from build123d import *

# Parameters (mm, degrees)
Y_KSEKLIK_EKSTR_ZYON1_DEPTH = 45
IZIM2_R                     = 30
KES_EKSTR_ZYON2_DEPTH       = 45


with BuildPart() as part:
    # Çizim1 → Yükseklik-Ekstrüzyon1 (new body)
    with BuildSketch(Plane(origin=(0, 0, 0), x_dir=(0, 0, -1), z_dir=(1, 0, 0))):
        with BuildLine():
            Line((-123, 75), (123, 75))
            ThreePointArc((123, 75), (142.091883092, 67.091883092), (150, 48))
            Line((150, 48), (150, -48))
            ThreePointArc((150, -48), (142.091883092, -67.091883092), (123, -75))
            Line((123, -75), (-123, -75))
            ThreePointArc((-123, -75), (-142.091883092, -67.091883092), (-150, -48))
            Line((-150, -48), (-150, 48))
            ThreePointArc((-150, 48), (-142.091883092, 67.091883092), (-123, 75))
        make_face()
    extrude(amount=Y_KSEKLIK_EKSTR_ZYON1_DEPTH)

    # Çizim2 → Kes-Ekstrüzyon2 (cut)
    with BuildSketch(Plane(origin=(45, 0, 0), x_dir=(0, 0, -1), z_dir=(1, 0, 0))):
        with Locations((100, -2.634150603)):
            Circle(IZIM2_R)
        with Locations((-100, 0)):
            Circle(IZIM2_R)
    extrude(amount=-KES_EKSTR_ZYON2_DEPTH, mode=Mode.SUBTRACT)


solid = part.part
Input: part model. Units: mm. Frame: model coordinates. Coordinates: 2 decimals unless noted, no trailing zeros. Loops run counter-clockwise (first coordinate to the right, second up) from the corner with the lowest first, then second, coordinate; pieces in that order, holes last. Notation, with made-up numbers: (1.5, -32) - (20.5, -32) arc R14 cw to (20.5, -8) - close; hole circle Ø3 at (49.5, 28). An arc over 180 degrees is marked (long way). Answer in a Markdown table with one row per item. Add a question column.
Item 1: Section query A-A on z = -100. Return the cut outline in (x, y).
Item 2: Mould query, pull axis Z, two halves, no side actions, for faces 1 (the cylindrical face through (22.82, 1.32, 129.97)), 2 (the cylindrical face through (22.18, 67.3, -141.88)), 3 (the cylindrical face through (22.18, 66.88, 142.3)), 4 (the cylindrical face through (22.82, -1.32, -70.03)). Classes: released by +Z, released by -Z, zero draft, split by the parting line, or undercut.
Item 3: Section query C-C on z = 92. Return the cut outline in (x, y), then the cut area to 3 significant figures.
Item 4: Section query D-D on y = 59.5. Return the cut outline in (x, z).
Item 5: Section query B-B on x = 36. Return the cut outline in (y, z), then the cut area to 3 significant figures.
Item 6: Line query: line 1 along Z through (x, y) = (35.5, -1); line 2 along Y through (x, z) = (17.5, -100); line 3 along Y through (x, z) = (21, 100). Output: solid intervals per line, ascending. Write a range as [from, to].
Recorded:
| question | item | result |
|---|---|---|
| 1 | outline | (0, -75) - (45, -75) - (45, -32.63) - (0, -32.63) - close; (0, 27.37) - (45, 27.37) - (45, 75) - (0, 75) - close |
| 2 | face 1 | undercut |
| 2 | face 2 | released by -Z |
| 2 | face 3 | released by +Z |
| 2 | face 4 | undercut |
| 3 | outline | (0, -75) - (45, -75) - (45, -28.91) - (0, -28.91) - close; (0, 28.91) - (45, 28.91) - (45, 75) - (0, 75) - close |
| 3 | area | 4,150 mm^2 |
| 4 | outline | (0, -147.43) - (45, -147.43) - (45, 147.43) - (0, 147.43) - close |
| 5 | outline | (-75, -123) arc R27 ccw to (-48, -150) - (48, -150) arc R27 ccw to (75, -123) - (75, 123) arc R27 ccw to (48, 150) - (-48, 150) arc R27 ccw to (-75, 123) - close; hole circle Ø60 at (-2.63, -100); hole circle Ø60 at (0, 100) |
| 5 | area | 38,700 mm^2 |
| 6 | line 1 | [-150, -129.96], [-70.04, 70.02], [129.98, 150] |
| 6 | line 2 | [-75, -32.63], [27.37, 75] |
| 6 | line 3 | [-75, -30], [30, 75] |
